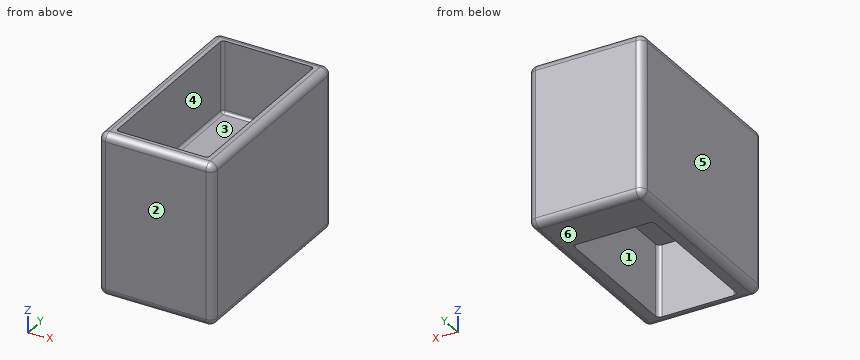
from build123d import *

# Parameters (mm, degrees)
F0_W     = 22.4
F0_H     = 40.2
F1_DEPTH = 25
F2_DEPTH = 20
F0_W_2   = 32
F0_H_2   = 56.1
F3_DEPTH = 45
F4_DEPTH = 20
F5_R     = 2
F6_R     = 0.8
F7_R     = 1.2


with BuildPart() as f1:
    # F0 (on Top) → F1 (new body)
    with BuildSketch(Plane.XY):
        Polygon((-11.2, -25.05), (-11.2, 15.15), (11.2, 15.15), (11.2, -25.05), (12.8, -25.05), (12.8, 25.05), (-12.8, 25.05), (-12.8, -25.05), align=None)
        with Locations((0, -4.95)):
            Rectangle(F0_W, F0_H)
    extrude(amount=F1_DEPTH)

    # F0 (on Top) → F2 (cut)
    with BuildSketch(Plane.XY):
        with Locations((0, -4.95)):
            Rectangle(F0_W, F0_H)
        Polygon((-11.2, -25.05), (-11.2, 15.15), (11.2, 15.15), (11.2, -25.05), (12.8, -25.05), (12.8, 25.05), (-12.8, 25.05), (-12.8, -25.05), align=None)
    extrude(amount=F2_DEPTH, mode=Mode.SUBTRACT)

    # F0 (on Top) → F3 (join)
    with BuildSketch(Plane.XY):
        Rectangle(F0_W_2, F0_H_2)
        Polygon((11.2, -25.05), (-11.2, -25.05), (-12.8, -25.05), (-12.8, 25.05), (12.8, 25.05), (12.8, -25.05), align=None, mode=Mode.SUBTRACT)
    extrude(amount=F3_DEPTH)

    # F0 (on Top) → F4 (join)
    with BuildSketch(Plane.XY):
        Polygon((-11.2, -25.05), (-11.2, 15.15), (11.2, 15.15), (11.2, -25.05), (12.8, -25.05), (12.8, 25.05), (-12.8, 25.05), (-12.8, -25.05), align=None)
    extrude(amount=F4_DEPTH)

    # F5
    f5_edges = [f1.edges().sort_by_distance(p)[0] for p in [
        (16, -28.05, 22.5),
        (16, 28.05, 22.5),
        (16, 0, 0),
        (16, 0, 45),
        (-16, 28.05, 22.5),
        (-16, -28.05, 22.5),
        (-16, 0, 0),
        (-16, 0, 45),
        (0, 28.05, 0),
        (0, 28.05, 45),
        (0, -28.05, 0),
        (0, -28.05, 45),
    ]]
    fillet(f5_edges, radius=F5_R)

    # F6
    f6_edges = [f1.edges().sort_by_distance(p)[0] for p in [
        (12.8, 25.05, 35),
        (12.8, -25.05, 35),
        (-12.8, -25.05, 35),
        (-12.8, 25.05, 35),
        (12.8, 0, 25),
        (0, 25.05, 25),
        (-12.8, 0, 25),
        (0, -25.05, 25),
    ]]
    fillet(f6_edges, radius=F6_R)

    # F7
    f7_edges = [f1.edges().sort_by_distance(p)[0] for p in [
        (-11.2, -25.05, 10),
        (11.2, -25.05, 10),
        (11.2, 15.15, 10),
        (-11.2, 15.15, 10),
    ]]
    fillet(f7_edges, radius=F7_R)


solid = f1.part
The model under review builds one solid part; all positions refer to its coordinate system, in mm. Face numbers are marked on the shaded views. A direction names the side the tool comes from. Coordinates: 2 decimals unless noted, no trailing zeros. Write each loop counter-clockwise with the first axis right and the second up, starting at its lowest first coordinate (ties: lowest second). Pieces come first, ordered by that corner, then holes. Notation, with made-up numbers: (18, -8.5) -> (60, -8.5) arc R17 ccw to (60, 0.5) -> close; hole circle Ø11 at (-29.5, 89.25). An arc over 180 degrees is marked (long way). Answer in a Markdown table with one row per item.
1. Draft analysis for pull direction X (two halves, no side actions). For the marked faces 4, 5 and 6, state which applies: +X half, -X half, draft (parallel to the pull), parting line (faces both ways), or undercut.
Answers below:
| item | result |
|---|---|
| face 4 | undercut |
| face 5 | -X half |
| face 6 | draft |
2. We need section D-D, the plane z = 10. State the section outline as (x, y) points, and give its area (3 significant figures).
Answers below:
| item | result |
|---|---|
| outline | (-16, -26.05) arc R2 ccw to (-14, -28.05) -> (14, -28.05) arc R2 ccw to (16, -26.05) -> (16, 26.05) arc R2 ccw to (14, 28.05) -> (-14, 28.05) arc R2 ccw to (-16, 26.05) -> close; hole (-11.2, -23.85) arc R1.2 ccw to (-10, -25.05) -> (10, -25.05) arc R1.2 ccw to (11.2, -23.85) -> (11.2, 13.95) arc R1.2 ccw to (10, 15.15) -> (-10, 15.15) arc R1.2 ccw to (-11.2, 13.95) -> close |
| area | 893 mm^2 |
3. Wall thickness on probe 1 along Y at (x, z) = (3, 13); probe 2 along X at (y, z) = (-22, 29.5); probe 3 along X at (y, z) = (-15.5, 14): over which ranges is each line inside the solid? List them lowest first. Write a range as [from, to].
Answers below:
| item | result |
|---|---|
| probe 1 | y = [-28.05, -25.05], [15.15, 28.05] |
| probe 2 | x = [-16, -12.8], [12.8, 16] |
| probe 3 | x = [-16, -11.2], [11.2, 16] |
4. We need section A-A, the plane z = 32.5. State the section outline as (x, y) points.
Answers below:
| item | result |
|---|---|
| outline | (-16, -26.05) arc R2 ccw to (-14, -28.05) -> (14, -28.05) arc R2 ccw to (16, -26.05) -> (16, 26.05) arc R2 ccw to (14, 28.05) -> (-14, 28.05) arc R2 ccw to (-16, 26.05) -> close; hole (-12.8, -24.25) arc R0.8 ccw to (-12, -25.05) -> (12, -25.05) arc R0.8 ccw to (12.8, -24.25) -> (12.8, 24.25) arc R0.8 ccw to (12, 25.05) -> (-12, 25.05) arc R0.8 ccw to (-12.8, 24.25) -> close |
5. We need section C-C, the plane x = -6.5. State the section outline as (y, z) points, and give its area (3 significant figures).
Answers below:
| item | result |
|---|---|
| outline | (-28.05, 2) arc R2 ccw to (-26.05, 0) -> (-25.05, 0) -> (-25.05, 20) -> (15.15, 20) -> (15.15, 0) -> (26.05, 0) arc R2 ccw to (28.05, 2) -> (28.05, 43) arc R2 ccw to (26.05, 45) -> (25.05, 45) -> (25.05, 25.8) arc R0.8 cw to (24.25, 25) -> (-24.25, 25) arc R0.8 cw to (-25.05, 25.8) -> (-25.05, 45) -> (-26.05, 45) arc R2 ccw to (-28.05, 43) -> close |
| area | 715 mm^2 |
6. Clearance check with flat-ended pins moving along their axes: pin 1 Ø19 at (x, y) = (0, 5.5) entering from +Z; pin 2 Ø6.5 at (x, y) = (3, -7.5) entering from -Z. State where each tip first meets the part, or that it passes through.
Answers below:
| item | result |
|---|---|
| pin 1 | stops at z = 25 |
| pin 2 | stops at z = 20 |
7. For the marked faces 1, 2 and 3, list the 3-axis set-ups (+Z, -Z, +X, -X, +Y, -Y) from which the entire face can be reached by the end or side of a thin tool; tool diameter is ignored.
Answers below:
| item | result |
|---|---|
| face 1 | -Z |
| face 2 | +Z, -Z, +X, -X, -Y |
| face 3 | +Z |
8. We need section B-B, the plane y = -19. State the section outline as (x, z) points.
Answers below:
| item | result |
|---|---|
| outline | (-16, 2) arc R2 ccw to (-14, 0) -> (-11.2, 0) -> (-11.2, 20) -> (11.2, 20) -> (11.2, 0) -> (14, 0) arc R2 ccw to (16, 2) -> (16, 43) arc R2 ccw to (14, 45) -> (12.8, 45) -> (12.8, 25.8) arc R0.8 cw to (12, 25) -> (-12, 25) arc R0.8 cw to (-12.8, 25.8) -> (-12.8, 45) -> (-14, 45) arc R2 ccw to (-16, 43) -> close |
